The model under review builds one solid part; all positions refer to its coordinate system, in mm. A direction names the side the tool comes from. Coordinates: 2 decimals unless noted, no trailing zeros. Loops run counter-clockwise (first coordinate to the right, second up) from the corner with the lowest first, then second, coordinate; pieces in that order, holes last. Notation, with made-up numbers: M 18,-27.75 L 50,-27.75 A19 cw 50,-18.75 Z; hole C -19.75,-1 d3. An arc over 180 degrees is marked long. Return JSON: item names as keys, results as strings.
```python
from build123d import *

# Parameters (mm, degrees)
BOSS_EXTRUDE1_DEPTH      = 6.35
CUT_EXTRUDE1_DEPTH       = 6.35
BOSS_EXTRUDE2_DEPTH      = 6.35
BOSS_EXTRUDE2_DEPTH_BACK = 12.7
SKETCH3_W                = 19.05
SKETCH3_H                = 6.35


with BuildPart() as part:
    # Sketch1 → Boss-Extrude1 (new body)
    with BuildSketch(Plane.XY):
        with BuildLine():
            Line((0, 0), (335.28, 0))
            Line((335.28, 0), (335.28, 313.51728))
            Line((335.28, 313.51728), (103.321320582, 313.51728))
            ThreePointArc((103.321320582, 313.51728), (87.853181888, 308.264157806), (78.783155215, 294.677648925))
            Line((78.783155215, 294.677648925), (0, 0))
        make_face()
    extrude(amount=BOSS_EXTRUDE1_DEPTH)

    # Sketch2 → Cut-Extrude1 (cut)
    with BuildSketch(Plane.XY.offset(6.35)):
        with BuildLine():
            Line((311.705446202, 12.7), (231.854553798, 12.7))
            ThreePointArc((231.854553798, 12.7), (224.165083065, 15.885083065), (220.98, 23.574553798))
            Line((220.98, 23.574553798), (220.98, 116.125446202))
            ThreePointArc((220.98, 116.125446202), (224.165083065, 123.814916935), (231.854553798, 127))
            Line((231.854553798, 127), (311.705446202, 127))
            ThreePointArc((311.705446202, 127), (319.394916935, 123.814916935), (322.58, 116.125446202))
            Line((322.58, 116.125446202), (322.58, 23.574553798))
            ThreePointArc((322.58, 23.574553798), (319.394916935, 15.885083065), (311.705446202, 12.7))
        make_face()
        with BuildLine():
            Line((203.603317785, 23.574553798), (203.603317785, 116.125446202))
            ThreePointArc((203.603317785, 116.125446202), (200.41823472, 123.814916935), (192.728763987, 127))
            Line((192.728763987, 127), (112.877871584, 127))
            ThreePointArc((112.877871584, 127), (105.18840085, 123.814916935), (102.003317785, 116.125446202))
            Line((102.003317785, 116.125446202), (102.003317785, 23.574553798))
            ThreePointArc((102.003317785, 23.574553798), (105.18840085, 15.885083065), (112.877871584, 12.7))
            Line((112.877871584, 12.7), (192.728763987, 12.7))
            ThreePointArc((192.728763987, 12.7), (200.41823472, 15.885083065), (203.603317785, 23.574553798))
        make_face()
        with BuildLine():
            Line((84.62663557, 23.574553798), (84.62663557, 116.125446202))
            ThreePointArc((84.62663557, 116.125446202), (81.441552505, 123.814916935), (73.752081772, 127))
            Line((73.752081772, 127), (59.157987156, 127))
            ThreePointArc((59.157987156, 127), (52.535581392, 124.750970083), (48.652412376, 118.934150328))
            Line((48.652412376, 118.934150328), (23.908590277, 26.383257925))
            ThreePointArc((23.908590277, 26.383257925), (25.788641176, 16.952148035), (34.414165057, 12.7))
            Line((34.414165057, 12.7), (73.752081772, 12.7))
            ThreePointArc((73.752081772, 12.7), (81.441552505, 15.885083065), (84.62663557, 23.574553798))
        make_face()
        with BuildLine():
            Line((203.603317785, 153.114553798), (203.603317785, 245.665446202))
            ThreePointArc((203.603317785, 245.665446202), (200.41823472, 253.354916935), (192.728763987, 256.54))
            Line((192.728763987, 256.54), (112.877871584, 256.54))
            ThreePointArc((112.877871584, 256.54), (105.18840085, 253.354916935), (102.003317785, 245.665446202))
            Line((102.003317785, 245.665446202), (102.003317785, 153.114553798))
            ThreePointArc((102.003317785, 153.114553798), (105.18840085, 145.425083065), (112.877871584, 142.24))
            Line((112.877871584, 142.24), (192.728763987, 142.24))
            ThreePointArc((192.728763987, 142.24), (200.41823472, 145.425083065), (203.603317785, 153.114553798))
        make_face()
        with BuildLine():
            Line((322.58, 153.114553798), (322.58, 245.665446202))
            ThreePointArc((322.58, 245.665446202), (319.394916935, 253.354916935), (311.705446202, 256.54))
            Line((311.705446202, 256.54), (231.854553798, 256.54))
            ThreePointArc((231.854553798, 256.54), (224.165083065, 253.354916935), (220.98, 245.665446202))
            Line((220.98, 245.665446202), (220.98, 153.114553798))
            ThreePointArc((220.98, 153.114553798), (224.165083065, 145.425083065), (231.854553798, 142.24))
            Line((231.854553798, 142.24), (311.705446202, 142.24))
            ThreePointArc((311.705446202, 142.24), (319.394916935, 145.425083065), (322.58, 153.114553798))
        make_face()
    extrude(amount=-CUT_EXTRUDE1_DEPTH, mode=Mode.SUBTRACT)

    # Sketch3 → Boss-Extrude2 (add, two sides: drawn at the far end of the back side and taken through both)
    with BuildSketch(Plane.XY.offset(6.35).offset(-BOSS_EXTRUDE2_DEPTH_BACK)):
        Polygon((11.43, -6.35), (11.43, 0), (0, 0), (-7.62, 0), (-7.62, -6.35), align=None)
        with Locations((40.005, -3.175)):
            Rectangle(SKETCH3_W, SKETCH3_H)
        with Locations((78.105, -3.175)):
            Rectangle(SKETCH3_W, SKETCH3_H)
        with Locations((116.205, -3.175)):
            Rectangle(SKETCH3_W, SKETCH3_H)
        with Locations((154.305, -3.175)):
            Rectangle(SKETCH3_W, SKETCH3_H)
        with Locations((192.405, -3.175)):
            Rectangle(SKETCH3_W, SKETCH3_H)
        with Locations((230.505, -3.175)):
            Rectangle(SKETCH3_W, SKETCH3_H)
        with Locations((268.605, -3.175)):
            Rectangle(SKETCH3_W, SKETCH3_H)
        with Locations((306.705, -3.175)):
            Rectangle(SKETCH3_W, SKETCH3_H)
    extrude(amount=BOSS_EXTRUDE2_DEPTH + BOSS_EXTRUDE2_DEPTH_BACK)


solid = part.part
```
1. Add section A-A on x = 283. Give the boundary of the cut face in (y, z), plus the area to 3 significant figures.
Check values:
{"outline": "M 0,0 L 12.7,0 L 12.7,6.35 L 0,6.35 Z; M 127,0 L 142.24,0 L 142.24,6.35 L 127,6.35 Z; M 256.54,0 L 313.52,0 L 313.52,6.35 L 256.54,6.35 Z", "area": "539 mm²"}
2. Machinability: for faces 4 (the face through (268, -6.35, 3)), 5 (the face through (204, 169, 6.35)), 6 (the face through (25.704, 17.063, 3.219)), which of the approach directions +Z, -Z, +X, -X, +Y, -Y give a long, thin tool a straight path to every point of the face, cutting with its end or side? Answer none if there is none.
Check values:
{"face 4": "+Z, -Z, +X, -X, -Y", "face 5": "+Z, +X, -X, +Y", "face 6": "+Z, -Z"}
3. The part is to be moulded in two halves that separate along X. For faces 1 (the face through (2, -6.35, 3)), 2 (the face through (36.454, 73.307, 3.219)), 3 (the face through (88.039, 308.405, 3.131)), say which applies: released by +X, released by -X, zero draft, split by the parting line, or undercut.
Check values:
{"face 1": "zero draft", "face 2": "undercut", "face 3": "released by -X"}
4. Add section D-D on y = 189. Give the boundary of the cut face in (x, z), plus the area to 3 significant figures.
Check values:
{"outline": "M 50.53,0 L 102,0 L 102,6.35 L 50.53,6.35 Z; M 203.6,0 L 220.98,0 L 220.98,6.35 L 203.6,6.35 Z; M 322.58,0 L 335.28,0 L 335.28,6.35 L 322.58,6.35 Z", "area": "518 mm²"}
5. To check wall thickness, follow line 1 (Y direction, x = 124.5, z = 4.75); line 2 (X direction, y = 250, z = 6); line 3 (X direction, y = 118.5, z = 3.5). State the ranges of each line that lie inside material, in increasing order.
Check values:
{"line 1": "-6.35 to 12.7, 127 to 142.24, 256.54 to 313.52", "line 2": "66.84 to 102.9, 202.7 to 221.88, 321.68 to 335.28", "line 3": "31.68 to 48.54, 84.36 to 102.27, 203.34 to 221.24, 322.32 to 335.28"}
6. Add section C-C on z = 9.5. State how many separate pieces and enclosed holes the cut face has, plus the area to 3 significant figures.
Check values:
{"separate pieces": "9", "enclosed holes": "0", "area": "1,090 mm²"}
7. Add section B-B on y = 82. Give the boundary of the cut face in (x, z).
Check values:
{"outline": "M 21.92,0 L 38.78,0 L 38.78,6.35 L 21.92,6.35 Z; M 84.63,0 L 102,0 L 102,6.35 L 84.63,6.35 Z; M 203.6,0 L 220.98,0 L 220.98,6.35 L 203.6,6.35 Z; M 322.58,0 L 335.28,0 L 335.28,6.35 L 322.58,6.35 Z"}
8. Insertion check: pin 1 Ø5 at (x, z) = (263.5, -3) entering from +Y; pin 2 Ø5 at (y, z) = (-4.5, -1.5) entering from +X; pin 3 Ø3 at (y, z) = (153.5, -3) entering from -X; pin 4 Ø10 at (x, y) = (87.5, 207.5) entering from +Z. Each pin has a flat end and moves straight along its axis. Give the tip position at first contact, or say it passes through.
Check values:
{"pin 1": "y = 0", "pin 2": "x = 316.23", "pin 3": "through", "pin 4": "z = 6.35"}
